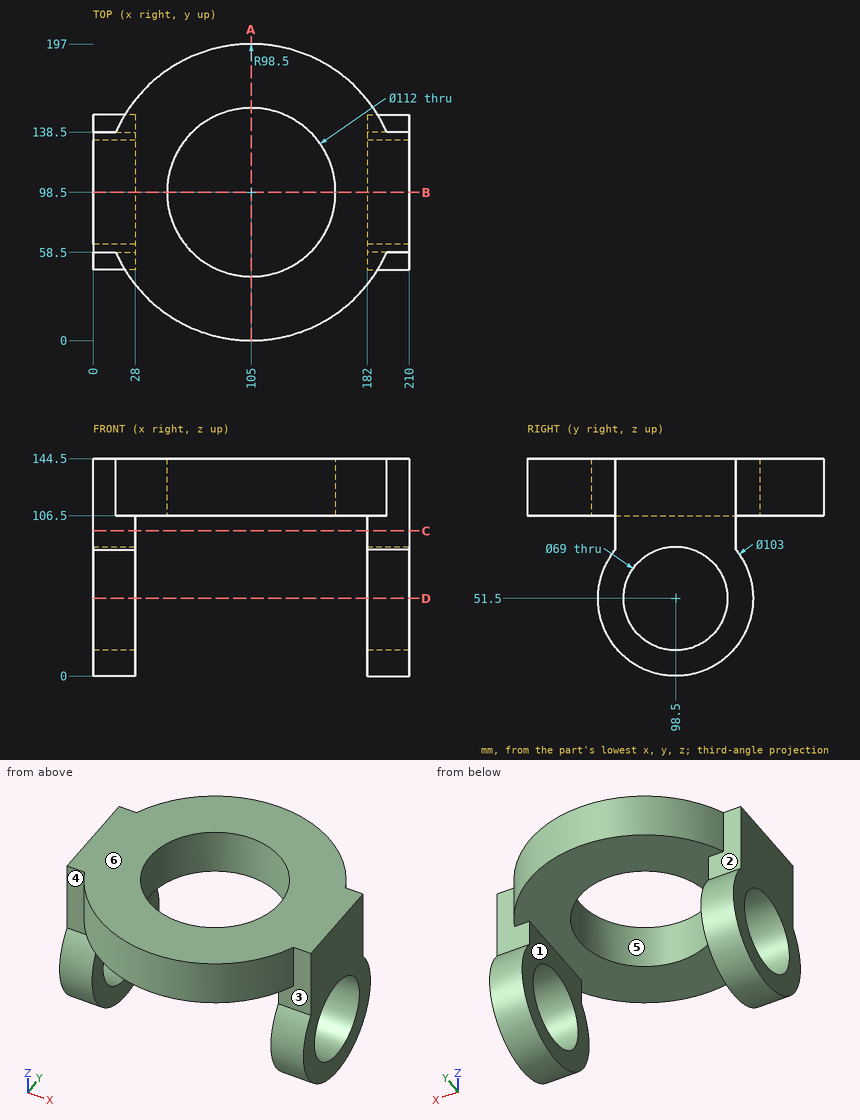
Input: dimensioned drawing with shaded views. Units: mm. Origin: part minimum x, y, z. A direction names the side the tool comes from. Coordinates: 2 decimals unless noted, no trailing zeros. Loops run counter-clockwise (first coordinate to the right, second up) from the corner with the lowest first, then second, coordinate; pieces in that order, holes last. Notation, with made-up numbers: M 82,82 L 92,82 A32 cw 92,115 Z; hole C 89,75.25 d4. An arc over 180 degrees is marked long. One line per item, written item: value. Start each with the question number.
1) Draft query along Z for the marked faces 4, 5 and 6. Return one class per face: released by +Z, released by -Z, zero draft, split by the parting line, or undercut.
2) Pin query (flat end, axial travel): P1, Ø8.5, axis at x = 200.5, z = 124.5, coming from the +Y side; P2, Ø8, axis at x = 54.5, y = 174, coming from the -Z side; P3, Ø8, axis at x = 173, z = 124.5, coming from the -Y side. Return the tip coordinate at first contact, or that it passes through.
3) Cut plane D-D (z = 51.5). Return loops of the section in (x, y), then the cut area to 3 significant figures.
4) Cut plane C-C (z = 96.5). Return loops of the section in (x, y), then the cut area to 3 significant figures.
5) Cut plane A-A (x = 105). Return loops of the section in (y, z).
6) Cut plane B-B (y = 98.5). Return loops of the section in (x, z), then the cut area to 3 significant figures.
7) Material intervals for L1, parallel to Y at x = 105, z = 121; L2, parallel to Z at x = 199, y = 98; L3, parallel to Z at x = 41, y = 29.5, sorted ascending. Write a range as from..to.
8) Reachability of the marked faces 1, 2 and 3 from +Z, -Z, +X, -X, +Y, -Y: full face, straight path, thin tool, end or side. Return the list, or none.
Evaluation:
1. face 4: undercut
1. face 5: zero draft
1. face 6: released by +Z
2. P1: y = 138.5
2. P2: z = 106.5
2. P3: y = 23.63
3. outline: M 0,47 L 28,47 L 28,64 L 0,64 Z; M 0,133 L 28,133 L 28,150 L 0,150 Z; M 182,47 L 210,47 L 210,64 L 182,64 Z; M 182,133 L 210,133 L 210,150 L 182,150 Z
3. area: 1,900 mm^2
4. outline: M 0,58.5 L 28,58.5 L 28,138.5 L 0,138.5 Z; M 182,58.5 L 210,58.5 L 210,138.5 L 182,138.5 Z
4. area: 4,480 mm^2
5. outline: M 0,106.5 L 42.5,106.5 L 42.5,144.5 L 0,144.5 Z; M 154.5,106.5 L 197,106.5 L 197,144.5 L 154.5,144.5 Z
6. outline: M 0,0 L 28,0 L 28,17 L 0,17 Z; M 0,86 L 28,86 L 28,106.5 L 49,106.5 L 49,144.5 L 0,144.5 Z; M 161,106.5 L 182,106.5 L 182,86 L 210,86 L 210,144.5 L 161,144.5 Z; M 182,0 L 210,0 L 210,17 L 182,17 Z
6. area: 5,820 mm^2
7. L1: 0..42.5, 154.5..197
7. L2: 0..17, 86..144.5
7. L3: 106.5..144.5
8. face 1: -Z, +Y, -Y
8. face 2: -X, +Y
8. face 3: +X, -Y
